Design review of the part built by this model. Coordinates are the model's own, in mm. Face numbers are marked on the shaded views. Coordinates: 2 decimals unless noted, no trailing zeros. Loops run counter-clockwise (first coordinate to the right, second up) from the corner with the lowest first, then second, coordinate; pieces in that order, holes last. Notation, with made-up numbers: (-40, 30) -> (16, 30) arc R8 ccw to (16, 40) -> close; hole circle Ø9 at (45, 18.5). An arc over 180 degrees is marked (long way). Use one line per item in the form item = value. Start each with the question number.
1. Consider section A-A (z = 1.9). State the section outline as (x, y) points, then the cut area to 3 significant figures.
2. Consider section B-B (y = 3.75). State the section outline as (x, z) points.
3. The part is to be moulded in two halves that separate along X. For the marked faces 1, 2 and 3, say which applies: released by +X, released by -X, zero draft, split by the parting line, or undercut.
4. Consider section C-C (x = 4). State the section outline as (y, z) points.
5. Wall thickness on line 1 (X direction, y = 10.5, z = 1.95); line 2 (Z direction, x = 8, y = 11): over which ranges is each line inside the solid? List them lowest first. Write a range as from..to.
Autodesk Inventor part; units mm, degrees
ref_plane "YZ Plane" through (0, 0, 0) normal (1, 0, 0) x (0, 1, 0)
ref_plane "XZ Plane" through (0, 0, 0) normal (0, 1, 0) x (-1, 0, 0)
ref_plane "XY Plane" through (0, 0, 0) normal (0, 0, 1) x (1, 0, 0)
sketch "Sketch1" plane through (0, 0, 0) normal (0, 0, 1) x (1, 0, 0)
  line L0 (0, 0) -> (20.32, 0)
  line L1 (20.32, 0) -> (20.32, 12.7)
  line L2 (20.32, 12.7) -> (0, 12.7)
  line L3 (0, 12.7) -> (0, 0)
  dimension "d0" = 20.32
  dimension "d1" = 12.7
extrude "Extrusion1" add sketch "Sketch1" along normal blind 1.27
sketch "Sketch2" plane through (0, 0, 1.27) normal (0, 0, 1) x (1, 0, 0)
  line L0 (20.32, 12.7) -> (0, 12.7)
  line L1 (0, 0) -> (1.016, 0)
  line L2 (1.016, 0) -> (1.016, 12.7)
  line L3 (1.016, 12.7) -> (0, 12.7)
  line L4 (0, 12.7) -> (0, 0)
  line L5 (20.32, 12.7) -> (19.304, 12.7)
  line L6 (19.304, 12.7) -> (19.304, 0)
  line L7 (19.304, 0) -> (20.32, 0)
  line L8 (20.32, 0) -> (20.32, 12.7)
  dimension "d4" = 1.016
  dimension "d5" = 1.016
extrude "Extrusion2" add sketch "Sketch2" along normal blind 1.27
properties part number "USBBreakoutCover"
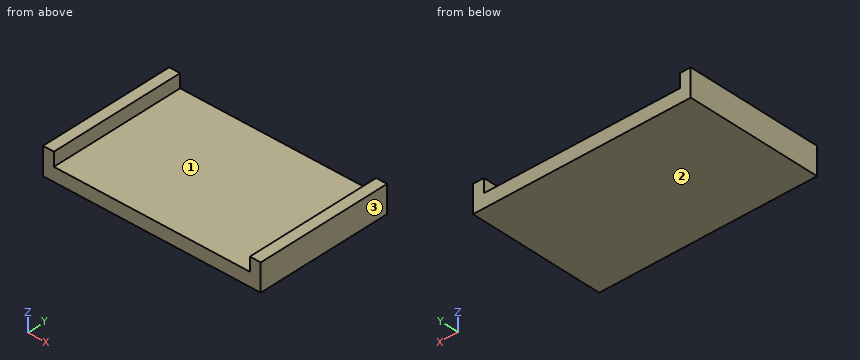
Geometry check:
q1.outline = (0, 0) -> (1.02, 0) -> (1.02, 12.7) -> (0, 12.7) -> close; (19.3, 0) -> (20.32, 0) -> (20.32, 12.7) -> (19.3, 12.7) -> close
q1.area = 25.8 mm²
q2.outline = (0, 0) -> (20.32, 0) -> (20.32, 2.54) -> (19.3, 2.54) -> (19.3, 1.27) -> (1.02, 1.27) -> (1.02, 2.54) -> (0, 2.54) -> close
q3.face_1 = undercut
q3.face_2 = zero draft
q3.face_3 = released by +X
q4.outline = (0, 0) -> (12.7, 0) -> (12.7, 1.27) -> (0, 1.27) -> close
q5.line_1 = 0..1.02, 19.3..20.32
q5.line_2 = 0..1.27
